The listing builds one solid part. Answer for the finished solid, in the listing's coordinates (mm). A direction names the side the tool comes from. Give positions to 0.01 mm unless a question says otherwise; leave off trailing zeros. Order: outer loops, then holes, each group sorted by start corner. A loop starts at its lowest first (then second) coordinate and runs counter-clockwise, first axis right, second up. Notation, with made-up numbers: (26, -35.75) -> (79, -35.75) arc R28 ccw to (79, -16.75) -> close; hole circle Ø1 at (7.25, 13.5). An arc over 180 degrees is marked (long way). One line per question, with ' | ' between items. Start each with the question number.
```python
from build123d import *

# Parameters (mm, degrees)
F1_DEPTH = 6.35


with BuildPart() as f1:
    # F0 (on Front) → F1 (new body)
    with BuildSketch(Plane.XZ):
        Polygon((38.1, 44.45), (38.1, 38.1), (31.75, 38.1), (31.75, 44.45), (25.4, 44.45), (25.4, 38.1), (19.05, 38.1), (19.05, 44.45), (12.7, 44.45), (12.7, 38.1), (6.35, 38.1), (6.35, 44.45), (0, 44.45), (0, 38.1), (-6.35, 38.1), (-6.35, 44.45), (-12.7, 44.45), (-12.7, 38.1), (-19.05, 38.1), (-19.05, 44.45), (-25.4, 44.45), (-25.4, 38.1), (-31.75, 38.1), (-31.75, 44.45), (-44.45, 44.45), (-44.45, 38.1), (-38.1, 38.1), (-38.1, 31.75), (-44.45, 31.75), (-44.45, 25.4), (-38.1, 25.4), (-38.1, 19.05), (-44.45, 19.05), (-44.45, 12.7), (-38.1, 12.7), (-38.1, 6.35), (-44.45, 6.35), (-44.45, 0), (-38.1, 0), (-38.1, -6.35), (-44.45, -6.35), (-44.45, -12.7), (-38.1, -12.7), (-38.1, -19.05), (-44.45, -19.05), (-44.45, -25.4), (-38.1, -25.4), (-38.1, -31.75), (-44.45, -31.75), (-44.45, -44.45), (-38.1, -44.45), (-38.1, -38.1), (-31.75, -38.1), (-31.75, -44.45), (-25.4, -44.45), (-25.4, -38.1), (-19.05, -38.1), (-19.05, -44.45), (-12.7, -44.45), (-12.7, -38.1), (-6.35, -38.1), (-6.35, -44.45), (0, -44.45), (0, -38.1), (6.35, -38.1), (6.35, -44.45), (12.7, -44.45), (12.7, -38.1), (19.05, -38.1), (19.05, -44.45), (25.4, -44.45), (25.4, -38.1), (31.75, -38.1), (31.75, -44.45), (44.45, -44.45), (44.45, -38.1), (38.1, -38.1), (38.1, -31.75), (44.45, -31.75), (44.45, -25.4), (38.1, -25.4), (38.1, -19.05), (44.45, -19.05), (44.45, -12.7), (38.1, -12.7), (38.1, -6.35), (44.45, -6.35), (44.45, 0), (38.1, 0), (38.1, 6.35), (44.45, 6.35), (44.45, 12.7), (38.1, 12.7), (38.1, 19.05), (44.45, 19.05), (44.45, 25.4), (38.1, 25.4), (38.1, 31.75), (44.45, 31.75), (44.45, 44.45), align=None)
    extrude(amount=F1_DEPTH)


solid = f1.part
```
(1) Given P1, Ø2, axis at x = 12.5, y = -2.5, coming from the +Z side; P2, Ø2, axis at x = 7.5, y = -3, coming from the +Z side; P3, Ø1.9, axis at y = -3.5, z = -36, coming from the +X side, each flat-ended and moving along its own axis, determine where each tip first touches the part or whether it passes through.
(2) Consider line 1 (Z direction, x = 11.5, y = -5.25); line 2 (Z direction, x = 14, y = -0.25). Determine where each line is inside the solid, lowest interval first.
(3) Determine the mould class of faces 1 (the face through (-19.05, -3, 41)), 2 (the face through (-16, -3, 38.1)), 3 (the face through (-41, -3, 25.4)) for opening direction Z: pulls with the +Z half, pulls with the -Z half, needs draft (parallel to the pull), parting line crosses it, or undercut.
(4) The part is cut by section B-B on x = -21. Determine the outline of the cut face in (y, z), plus the area to 3 significant figures.
(5) For faces 4 (the face through (-41, -3, -19.05)), 5 (the face through (41, -3, -12.7)), 6 (the face through (19.05, -3, 41)), determine the directions among +Z, -Z, +X, -X, +Y, -Y from which every point of the face is accessible in a straight line to the end or side of a thin tool.
(6) The part is cut by section A-A on z = 22. Determine the outline of the cut face in (x, y).
Result sheet:
1) P1: stops at z = 44.45 | P2: stops at z = 38.1 | P3: stops at x = 38.1
2) line 1: z = -44.45 to 38.1 | line 2: z = -38.1 to 44.45
3) face 1: needs draft | face 2: pulls with the +Z half | face 3: undercut
4) outline: (-6.35, -38.1) -> (0, -38.1) -> (0, 44.45) -> (-6.35, 44.45) -> close | area: 524 mm^2
5) face 4: -X, +Y, -Y | face 5: +X, +Y, -Y | face 6: +Z, +Y, -Y
6) outline: (-38.1, -6.35) -> (44.45, -6.35) -> (44.45, 0) -> (-38.1, 0) -> close
